from build123d import *

# Parameters (mm, degrees)
PAD_DEPTH   = 3
FILLET_R    = 0.8
FILLET001_R = 0.8
FILLET002_R = 0.5
FILLET003_R = 0.5
FILLET004_R = 1
FILLET005_R = 1


with BuildPart() as part:
    # Sketch → Pad (new body)
    with BuildSketch(Plane.XY):
        Polygon((-4, 0), (-6, 0), (-6, 4), (6, 4), (6, 0), (4, 0), (4, 2.48), (-4, 2.48), align=None)
    extrude(amount=PAD_DEPTH)

    # Fillet
    fillet_edges = [part.edges().sort_by_distance(p)[0] for p in [
        (0, 4, 3),
    ]]
    fillet(fillet_edges, radius=FILLET_R)

    # Fillet001
    fillet001_edges = [part.edges().sort_by_distance(p)[0] for p in [
        (0, 4, 0),
    ]]
    fillet(fillet001_edges, radius=FILLET001_R)

    # Fillet002
    fillet002_edges = [part.edges().sort_by_distance(p)[0] for p in [
        (6, 1.6, 3),
    ]]
    fillet(fillet002_edges, radius=FILLET002_R)

    # Fillet003
    fillet003_edges = [part.edges().sort_by_distance(p)[0] for p in [
        (-6, 1.6, 0),
    ]]
    fillet(fillet003_edges, radius=FILLET003_R)

    # Fillet004
    fillet004_edges = [part.edges().sort_by_distance(p)[0] for p in [
        (-4, 2.48, 1.5),
    ]]
    fillet(fillet004_edges, radius=FILLET004_R)

    # Fillet005
    fillet005_edges = [part.edges().sort_by_distance(p)[0] for p in [
        (4, 2.48, 1.5),
    ]]
    fillet(fillet005_edges, radius=FILLET005_R)


solid = part.part
CAD build for the part. Positions are in the model's coordinates, mm. A direction names the side the tool comes from. Coordinates: 2 decimals unless noted, no trailing zeros. Order: outer loops, then holes, each group sorted by start corner. A loop starts at its lowest first (then second) coordinate and runs counter-clockwise, first axis right, second up. Notation, with made-up numbers: (0.25, 85.25) -> (22.25, 85.25) arc R28 ccw to (22.25, 122.25) -> close; hole circle Ø7 at (13, -30). An arc over 180 degrees is marked (long way). Answer in a Markdown table with one row per item.
1) Drill centre lines: line 1 (X direction, y = 0.2, z = 2.4); line 2 (Y direction, x = -1, z = 1.25); line 3 (X direction, y = 1.95, z = 1.5). Where is each one in solid material? Low to high.
Check values:
| item | result |
|---|---|
| line 1 | -6 to -4, 4 to 6 |
| line 2 | 2.48 to 4 |
| line 3 | -6 to -3.88, 3.88 to 6 |
2) Band-saw the part on C-C (x = 4.25). List the corners of the cut face in (y, z).
Check values:
| item | result |
|---|---|
| outline | (0, 0) -> (3.2, 0) arc R0.8 ccw to (4, 0.8) -> (4, 2.2) arc R0.8 ccw to (3.2, 3) -> (0, 3) -> close |
3) Band-saw the part on D-D (x = -2.5). List the corners of the cut face in (y, z), and give its area (3 significant figures).
Check values:
| item | result |
|---|---|
| outline | (2.48, 0) -> (3.2, 0) arc R0.8 ccw to (4, 0.8) -> (4, 2.2) arc R0.8 ccw to (3.2, 3) -> (2.48, 3) -> close |
| area | 4.29 mm2 |
4) Band-saw the part on A-A (y = 2.1). List the corners of the cut face in (x, z).
Check values:
| item | result |
|---|---|
| outline | (-6, 0.5) arc R0.5 ccw to (-5.5, 0) -> (-3.78, 0) -> (-3.78, 3) -> (-5.5, 3) arc R0.5 ccw to (-6, 2.5) -> close; (3.78, 0) -> (5.5, 0) arc R0.5 ccw to (6, 0.5) -> (6, 2.5) arc R0.5 ccw to (5.5, 3) -> (3.78, 3) -> close |
5) Band-saw the part on B-B (z = 1.5). List the corners of the cut face in (x, y), and give its area (3 significant figures).
Check values:
| item | result |
|---|---|
| outline | (-6, 0) -> (-4, 0) -> (-4, 1.48) arc R1 cw to (-3, 2.48) -> (3, 2.48) arc R1 cw to (4, 1.48) -> (4, 0) -> (6, 0) -> (6, 3.5) arc R0.5 ccw to (5.5, 4) -> (-5.5, 4) arc R0.5 ccw to (-6, 3.5) -> close |
| area | 28.5 mm2 |
6) Which spindle directions (+Z, -Z, +X, -X, +Y, -Y) get a long thin tool onto all of the face, cutting with end or side? Do faces 4 (the face through (0, 3, 3)), 5 (the face through (3.699, 2.195, 1.521)). Say none if no direction does.
Check values:
| item | result |
|---|---|
| face 4 | +Z, +X, -X, +Y, -Y |
| face 5 | +Z, -Z, -Y |
7) Mould opens along X. For faces 1 (the face through (0, 4, 1)), 2 (the face through (-6, 2, 1)), 3 (the face through (4, 1, 1)) say: pulls with the +X half, pulls with the -X half, needs draft (parallel to the pull), parting line crosses it, or undercut.
Check values:
| item | result |
|---|---|
| face 1 | needs draft |
| face 2 | pulls with the -X half |
| face 3 | undercut |
